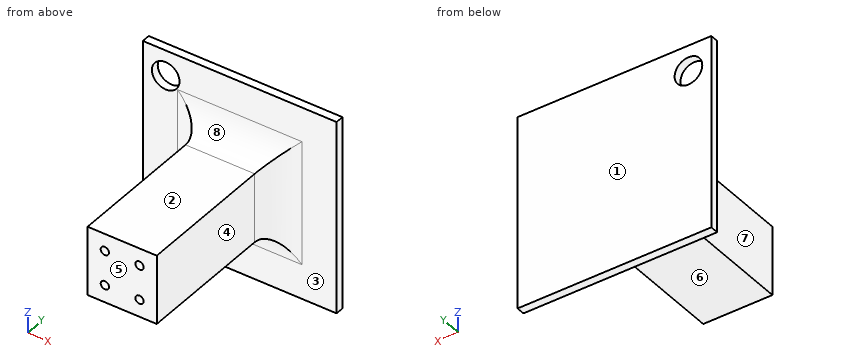
Autodesk Fusion 360 part; units mm, degrees
sketch "Sketch1" plane through (0, 0, 0) normal (0, 1, 0) x (1, 0, 0)
  line L0 (0, 0) -> (25, 0)
  line L1 (25, 0) -> (25, -25)
  line L2 (25, -25) -> (0, -25)
  line L3 (0, -25) -> (0, 0)
  dimension "d1" = 25
  dimension "d2" = 25
extrude "Extrude1" add sketch "Sketch1" along normal blind 60
sketch "Sketch2" plane through (0, 60, 0) normal (0, 1, 0) x (-1, 0, 0)
  line L0 (0, 25) -> (-25, 25)
  line L1 (-25, 25) -> (-25, 0)
  line L2 (-25, 0) -> (0, 0)
  line L3 (0, 0) -> (0, 25)
  line L4 (-47.5, 47.5) -> (22.5, 47.5)
  line L5 (22.5, 47.5) -> (22.5, -22.5)
  line L6 (22.5, -22.5) -> (-47.5, -22.5)
  line L7 (-47.5, -22.5) -> (-47.5, 47.5)
  line L8 (-47.5, 47.5) -> (22.5, -22.5) construction
  line L9 (22.5, 47.5) -> (-47.5, -22.5) construction
  point P0 (-12.5, 12.5)
  dimension "d5" = 70
  dimension "d6" = 70
extrude "Extrude2" add sketch "Sketch2" along normal blind 3 contours L0 L1 L2 L3 | L4 L5 L6 L7
fillet "Fillet1" radius 10 4 edges at (12.5, 60, 25) (25, 60, 12.5) (0, 60, 12.5) (12.5, 60, 0)
sketch "Sketch3" plane through (0, 63, 0) normal (0, 1, 0) x (-1, 0, 0)
  line L0 (-47.5, -22.5) -> (22.5, -22.5)
  line L1 (22.5, -22.5) -> (22.5, 47.5)
  line L2 (22.5, 47.5) -> (-47.5, 47.5)
  line L3 (-47.5, 47.5) -> (-47.5, -22.5)
  circle A0 centre (14.2428, 38.2388) radius 5
  dimension "d11" = 10
extrude "Extrude3" cut sketch "Sketch3" against normal blind 30 contours A0
sketch "Sketch4" plane through (0, 0, 0) normal (0, 1, 0) x (1, 0, 0)
  line L0 (25, 0) -> (0, 0)
  line L1 (0, 0) -> (0, -25)
  line L2 (0, -25) -> (25, -25)
  line L3 (25, -25) -> (25, 0)
  circle A0 centre (18.75, -6.25) radius 1.5
  circle A1 centre (18.767, -18.75) radius 1.5
  circle A2 centre (6.25, -6.25) radius 1.5
  circle A3 centre (6.233, -18.75) radius 1.5
  point P0 (25, 0)
  point P1 (25, -25)
  dimension "d14" = 3
  dimension "d15" = 3
  dimension "d17" = 12.5
  dimension "d18" = 6.25
extrude "Extrude4" cut sketch "Sketch4" along normal blind 7 contours A0 | A1 | A2 | A3
equation "d17 = 2.5 / 2 * 1 cm"
equation "d18 = 2.5 / 4 * 1 cm"
The model under review builds one solid part; all positions refer to its coordinate system, in mm. Face numbers are marked on the shaded views. A direction names the side the tool comes from. Round coordinates to 2 decimals unless told otherwise and drop trailing zeros. Write each loop counter-clockwise with the first axis right and the second up, starting at its lowest first coordinate (ties: lowest second). Pieces come first, ordered by that corner, then holes.
(1) We need section D-D on z = 21.5. Give the boundary of the cut face in (x, y), and give its area (3 significant figures).
(2) Insertion check: pin 1 (3 mm diameter, centred on x = 29.5, z = -11, fed in from -Y); pin 2 (1.5 mm diameter, centred on x = 3.5, y = 27, fed in from +Z); pin 3 (12 mm diameter, centred on y = 52, z = -13.5, fed in from +X); pin 4 (2.5 mm diameter, centred on x = 6.25, z = 6.25, fed in from -Y). Each pin has a flat end and moves straight along its axis. Give the tip position at first contact, or say it passes through.
(3) Mouldability with a two-part tool opening along Y and no side actions: class the marked faces 1, 2 and 3 as +Y half, -Y half, draft (parallel to the pull), parting line (faces both ways), or undercut.
(4) We need section C-C on x = 2. Give the boundary of the cut face in (y, z), and give its area (3 significant figures).
(5) Machinability: for the marked faces 4, 5, 6, 7 and 8, which of the approach directions +Z, -Z, +X, -X, +Y, -Y give a long, thin tool a straight path to every point of the face, cutting with its end or side? Answer none if there is none.
(6) We need section A-A on y = 5. Give the boundary of the cut face in (x, z), and give its area (3 significant figures).
(7) We need section B-B on z = 36. Give the boundary of the cut face in (x, y), and give its area (3 significant figures).
(8) Wall thickness on L1, parallel to Z at x = 6, y = 3; L2, parallel to X at y = 5.75, z = 18.75: over which ranges is each line inside the solid? List them lowest first.
Findings below:
1. outline: (-22.5, 60) - (-10, 60) arc R10 cw to (0, 50) - (0, 0) - (25, 0) - (25, 50) arc R10 cw to (35, 60) - (47.5, 60) - (47.5, 63) - (-22.5, 63) - close
1. area: 1,750 mm2
2. pin 1: stops at y = 59.99
2. pin 2: stops at z = 25
2. pin 3: passes through
2. pin 4: stops at y = 7
3. face 1: +Y half
3. face 2: draft
3. face 3: -Y half
4. outline: (0, 0) - (50, 0) arc R10 cw to (60, -10) - (60, -22.5) - (63, -22.5) - (63, 47.5) - (60, 47.5) - (60, 35) arc R10 cw to (50, 25) - (0, 25) - close
4. area: 1,750 mm2
5. face 4: +Z, -Z, +X, -Y
5. face 5: +Z, -Z, +X, -X, -Y
5. face 6: -Z, +X, -X, -Y
5. face 7: +Z, -Z, -X, -Y
5. face 8: +Z, +X, -X, -Y
6. outline: (0, 0) - (25, 0) - (25, 25) - (0, 25) - close; hole circle Ø3 at (6.23, 18.75); hole circle Ø3 at (6.25, 6.25); hole circle Ø3 at (18.75, 6.25); hole circle Ø3 at (18.77, 18.75)
6. area: 597 mm2
7. outline: (-22.5, 60) - (-18.71, 60) - (-18.71, 63) - (-22.5, 63) - close; (-9.77, 60) - (47.5, 60) - (47.5, 63) - (-9.77, 63) - close
7. area: 183 mm2
8. L1: z = 0 to 4.77, 7.73 to 17.27, 20.23 to 25
8. L2: x = 0 to 4.73, 7.73 to 17.27, 20.27 to 25
